```python
from build123d import *

# Parameters (mm, degrees)
F1_DEPTH = 19.05
F2_R     = 18.796
F3_DEPTH = 19.051
F5_DEPTH = 19.051


with BuildPart() as f1:
    # F0 (on Top) → F1 (new body)
    with BuildSketch(Plane.XY):
        with BuildLine():
            ThreePointArc((114.3, 25.4), (106.860512, 43.360512), (88.9, 50.8))
            Line((88.9, 50.8), (-88.9, 50.8))
            ThreePointArc((-88.9, 50.8), (-106.860512, 43.360512), (-114.3, 25.4))
            Line((-114.3, 25.4), (-114.3, -25.4))
            ThreePointArc((-114.3, -25.4), (-106.860512, -43.360512), (-88.9, -50.8))
            Line((-88.9, -50.8), (88.9, -50.8))
            ThreePointArc((88.9, -50.8), (106.860512, -43.360512), (114.3, -25.4))
            Line((114.3, -25.4), (114.3, 25.4))
        make_face()
    extrude(amount=F1_DEPTH)

    # F2 (on face) → F3 (cut, through all)
    with BuildSketch(Plane.XY.offset(19.05)):
        Circle(F2_R)
    extrude(amount=-F3_DEPTH, mode=Mode.SUBTRACT)

    # F4 (on face) → F5 (cut, through all)
    with BuildSketch(Plane.XY.offset(19.05)):
        with BuildLine():
            Line((-48.006, -50.8), (-48.006, -5.406457))
            ThreePointArc((-48.006, -5.406457), (-68.58, 21.2725), (-89.154, -5.406457))
            Line((-89.154, -5.406457), (-89.154, -50.8))
            Line((-89.154, -50.8), (-48.006, -50.8))
        make_face()
        with BuildLine():
            ThreePointArc((48.006, 5.406457), (68.58, -21.2725), (89.154, 5.406457))
            Line((89.154, 5.406457), (89.154, 50.8))
            Line((89.154, 50.8), (48.006, 50.8))
            Line((48.006, 50.8), (48.006, 5.406457))
        make_face()
    extrude(amount=-F5_DEPTH, mode=Mode.SUBTRACT)


solid = f1.part
```
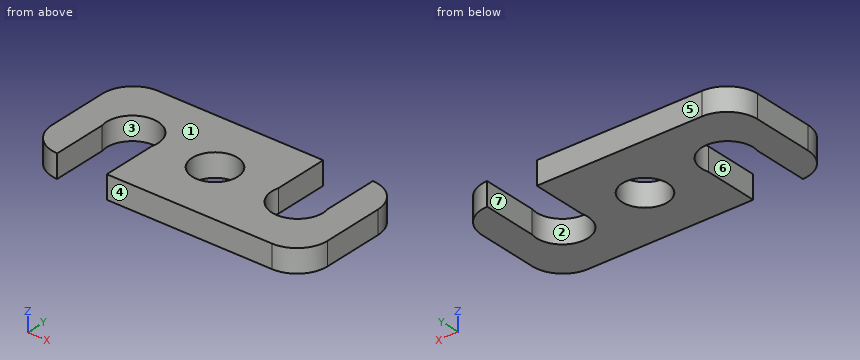
Build history of the part. All positions in model axes, mm. Face numbers are marked on the shaded views. A direction names the side the tool comes from. Round coordinates to 2 decimals unless told otherwise and drop trailing zeros. Order: outer loops, then holes, each group sorted by start corner. A loop starts at its lowest first (then second) coordinate and runs counter-clockwise, first axis right, second up. Notation, with made-up numbers: (84, 79) -> (140, 79) arc R18 cw to (140, 96) -> close; hole circle Ø5 at (44, 47.25). An arc over 180 degrees is marked (long way). Answer in a Markdown table with one row per item.
1) Band-saw the part on C-C on z = 4.5. Give the cut face in (x, y) (1 decimal), and give its area (3 significant figures).
Values:
| item | result |
|---|---|
| outline | (-114.3, -25.4) arc R25.4 ccw to (-89.2, -50.8) -> (-89.2, -5.4) arc R21.3 cw (long way) to (-48, -5.4) -> (-48, -50.8) -> (88.9, -50.8) arc R25.4 ccw to (114.3, -25.4) -> (114.3, 25.4) arc R25.4 ccw to (89.2, 50.8) -> (89.2, 5.4) arc R21.3 cw (long way) to (48, 5.4) -> (48, 50.8) -> (-88.9, 50.8) arc R25.4 ccw to (-114.3, 25.4) -> close; hole circle Ø37.6 at (0, 0) |
| area | 15,900 mm2 |
2) Band-saw the part on D-D on y = -31. Give the cut face in (x, z), and give its area (3 significant figures).
Values:
| item | result |
|---|---|
| outline | (-113.67, 0) -> (-89.15, 0) -> (-89.15, 19.05) -> (-113.67, 19.05) -> close; (-48.01, 0) -> (113.67, 0) -> (113.67, 19.05) -> (-48.01, 19.05) -> close |
| area | 3,550 mm2 |
3) Band-saw the part on A-A on x = 0. Give the cut face in (y, z), and give its area (3 significant figures).
Values:
| item | result |
|---|---|
| outline | (-50.8, 0) -> (-18.8, 0) -> (-18.8, 19.05) -> (-50.8, 19.05) -> close; (18.8, 0) -> (50.8, 0) -> (50.8, 19.05) -> (18.8, 19.05) -> close |
| area | 1,220 mm2 |
4) Wall check: L1, parallel to X at y = 23.5, z = 9.25; L2, parallel to X at y = -9, z = 13; L3, parallel to X at y = -19.5, z = 15. Give the ranges that are in metal, low to high.
Values:
| item | result |
|---|---|
| L1 | -114.3 to 48.01, 89.15 to 114.3 |
| L2 | -114.3 to -89.15, -48.01 to -16.5, 16.5 to 49.31, 87.85 to 114.3 |
| L3 | -114.3 to -89.15, -48.01 to 60.08, 77.08 to 114.3 |
5) Pin check, flat tips, straight feed: P1, Ø9.5, axis at y = 38, z = 12.5, coming from the +X side; P2, Ø6, axis at x = -48.5, y = -16, coming from the +Z side; P3, Ø6, axis at y = -31, z = 12, coming from the -X side. Stop position of each tip, or through.
Values:
| item | result |
|---|---|
| P1 | x = 113.06 |
| P2 | z = 19.05 |
| P3 | x = -114.17 |
6) Which spindle directions (+Z, -Z, +X, -X, +Y, -Y) get a long thin tool onto all of the face, cutting with end or side? Do the marked faces 5, 6 and 7. Say none if no direction does.
Values:
| item | result |
|---|---|
| face 5 | +Z, -Z, +X, -X, +Y |
| face 6 | +Z, -Z, -Y |
| face 7 | +Z, -Z, +Y |
7) Band-saw the part on B-B on y = 0. Give the cut face in (x, z).
Values:
| item | result |
|---|---|
| outline | (-114.3, 0) -> (-89.85, 0) -> (-89.85, 19.05) -> (-114.3, 19.05) -> close; (-47.31, 0) -> (-18.8, 0) -> (-18.8, 19.05) -> (-47.31, 19.05) -> close; (18.8, 0) -> (47.31, 0) -> (47.31, 19.05) -> (18.8, 19.05) -> close; (89.85, 0) -> (114.3, 0) -> (114.3, 19.05) -> (89.85, 19.05) -> close |
8) Mould opens along Y. For the marked faces 1, 2, 3 and 4 say: released by +Y, released by -Y, zero draft, split by the parting line, or undercut.
Values:
| item | result |
|---|---|
| face 1 | zero draft |
| face 2 | undercut |
| face 3 | undercut |
| face 4 | released by -Y |
